Geometry check sheet. Reference: the model listing, model coordinates, mm. A direction names the side the tool comes from. Round coordinates to 2 decimals unless told otherwise and drop trailing zeros. Order: outer loops, then holes, each group sorted by start corner. A loop starts at its lowest first (then second) coordinate and runs counter-clockwise, first axis right, second up. Notation, with made-up numbers: M -30.75,67 L -9.75,67 A21 ccw -9.75,83 Z; hole C -3,19.5 d8. An arc over 180 degrees is marked long. Return JSON: item names as keys, results as strings. Group by question number.
```python
from build123d import *

# Parameters (mm, degrees)
F2_SIZE = 0.99999


# Not quite as in the source:
# - a fillet or chamfer is up to 0.001 mm smaller than in the source, because OpenCascade refuses the exact size


with BuildPart() as f1:
    # F0 (on Right) → F1 (revolve)
    with BuildSketch(Plane.YZ):
        Polygon((0, 5), (0, 0), (800, 0), (800, 5), (789, 5), (789, 8), (54, 8), (54, 6), (15, 6), (15, 5), align=None)
    revolve(axis=Axis((0, 344.1624132916, 0), (0, 1, 0)))

    # F2 (size 1 in the source; OpenCascade refuses exactly that, so slightly less here)
    f2_edges = [f1.edges().sort_by_distance(p)[0] for p in [
        (0, 0, -5),
        (0, 15, -6),
        (0, 800, -5),
    ]]
    chamfer(f2_edges, length=F2_SIZE)


solid = f1.part
```
Q1. Set-up check for faces 1 (the face through (6, 54, -2)), 2 (the face through (-7.81, 416.36, -1.73)), 3 (the face through (-5.2, 789, 0.1)): record each of +Z, -Z, +X, -X, +Y, -Y from which the full face is reachable in a straight line by a thin tool's end or side.
Q2. Section check C-C on y = 515. Record the cut outline in (x, z), plus the area to 3 significant figures.
Q3. Material ranges on line 1 along Z through (x, y) = (6.25, 662); line 2 along Y through (x, z) = (-4.5, 6); line 3 along Y through (x, z) = (-1, -5), recorded low to high.
Q4. Depth check by flat-ended pin: pin 1 Ø3 at (y, z) = (233, 5.5) entering from +X; pin 2 Ø6 at (y, z) = (417, 5) entering from +X; pin 3 Ø1.5 at (y, z) = (150.5, 6) entering from -X. Enter the tip coordinate at first touch or a pass-through.
Geometry check:
{
 "1": {"face 1": "-Y", "face 2": "+Y, -Y", "face 3": "+Y"},
 "2": {"outline": "C 0,0 d16", "area": "201 mm^2"},
 "3": {"line 1": "z = -4.99 to 4.99", "line 2": "y = 54 to 789", "line 3": "y = 15.1 to 789"},
 "4": {"pin 1": "stops at x = 6.93", "pin 2": "stops at x = 7.75", "pin 3": "stops at x = -6.04"}
}
